Check sheet for the modelled part. Datum: model origin and axes. Units: mm. Face numbers are marked on the shaded views. A direction names the side the tool comes from. Round coordinates to 2 decimals unless told otherwise and drop trailing zeros. Write each loop counter-clockwise with the first axis right and the second up, starting at its lowest first coordinate (ties: lowest second). Pieces come first, ordered by that corner, then holes.
Item 1: Cross-section at B-B on x = 0. Enter the section's corners in (y, z), plus the area to 3 significant figures.
Item 2: Go/stop test with a flat-tipped pin: pin 1 Ø1 at (y, z) = (5, 3) entering from +X. Record where the tip stops, or that it passes through.
Item 3: Tool access check on the marked faces 5 and 6. Record the directions out of +Z, -Z, +X, -X, +Y, -Y that give a thin tool (end or side, any length) a straight path to the whole face; none if there is none.
Item 4: Release check for a two-part mould opening along Y. For the marked faces 1, 2, 3 and 4 record: +Y half, -Y half, draft (parallel to the pull), parting line (faces both ways), or undercut.
Item 5: Cross-section at A-A on y = 0. Enter the section's corners in (x, z), plus the area to 3 significant figures.
Item 6: Material ranges on line 1 (Y direction, x = 0, z = 3.5); line 2 (Y direction, x = 1, z = 2.25); line 3 (X direction, y = -2, z = 3.5), recorded low to high.
Item 7: Cross-section at C-C on y = -26. Enter the section's corners in (x, z).
from build123d import *

# Parameters (mm, degrees)
SKETCH1_R           = 20.66925
BOSS_EXTRUDE1_DEPTH = 6.35


with BuildPart() as part:
    # Sketch1 → Boss-Extrude1 (new body)
    with BuildSketch(Plane.XY):
        with BuildLine():
            Line((-10.265793628, 35.791116693), (10.265793628, 35.791116693))
            Line((10.265793628, 35.791116693), (10.265793628, 29.50036983))
            add(Edge.make_bspline(
                [(30.787817782, 12.869231593), (24.871862383, 26.630631307), (10.265793628, 29.50036983)],
                knots=[0, 0, 0, 1, 1, 1], degree=2))
            ThreePointArc((30.787817782, 12.869231593), (0, -33.36925), (-30.787817782, 12.869231593))
            add(Edge.make_bspline(
                [(-30.787817782, 12.869231593), (-24.871862383, 26.630631307), (-10.265793628, 29.50036983)],
                knots=[0, 0, 0, 1, 1, 1], degree=2))
            Line((-10.265793628, 29.50036983), (-10.265793628, 35.791116693))
        make_face()
        Circle(SKETCH1_R, mode=Mode.SUBTRACT)
    extrude(amount=BOSS_EXTRUDE1_DEPTH)


solid = part.part
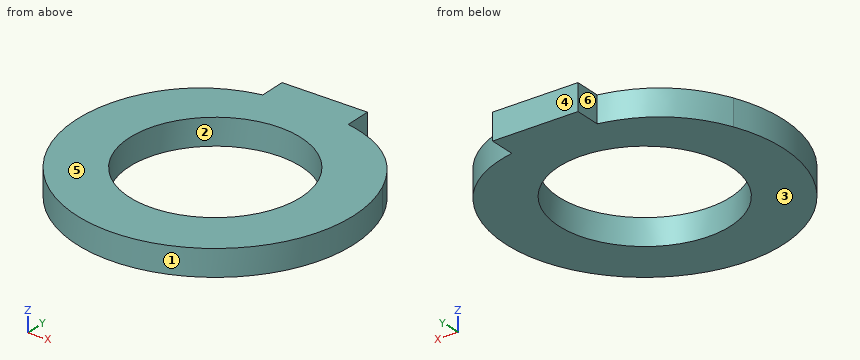
Response values:
1. outline: (-33.37, 0) - (-20.67, 0) - (-20.67, 6.35) - (-33.37, 6.35) - close; (20.67, 0) - (35.79, 0) - (35.79, 6.35) - (20.67, 6.35) - close
1. area: 177 mm2
2. pin 1: stops at x = 33.06
3. face 5: +Z, +X, -X, +Y, -Y
3. face 6: +Z, -Z, -X, +Y
4. face 1: parting line
4. face 2: undercut
4. face 3: draft
4. face 4: +Y half
5. outline: (-33.37, 0) - (-20.67, 0) - (-20.67, 6.35) - (-33.37, 6.35) - close; (20.67, 0) - (33.37, 0) - (33.37, 6.35) - (20.67, 6.35) - close
5. area: 161 mm2
6. line 1: y = -33.37 to -20.67, 20.67 to 35.79
6. line 2: y = -33.35 to -20.65, 20.65 to 35.79
6. line 3: x = -33.31 to -20.57, 20.57 to 33.31
7. outline: (-20.92, 0) - (20.92, 0) - (20.92, 6.35) - (-20.92, 6.35) - close
